Work out the finished part from the listing and answer in its coordinate system (mm). Round coordinates to 2 decimals unless told otherwise and drop trailing zeros. Loops run counter-clockwise (first coordinate to the right, second up) from the corner with the lowest first, then second, coordinate; pieces in that order, holes last. Notation, with made-up numbers: (69.25, 11.25) - (99.25, 11.25) arc R27 cw to (99.25, 27.25) - close; hole circle Ø7 at (76, 52). An arc over 180 degrees is marked (long way). Answer as CSV lines item,"result". Start each with the question number.
Q1. Section A-A on y = 7 is taken. Write down the section's boundary in (x, z), then the cut area to 3 significant figures.
Q2. This flat-tipped pin is pushed along its axis until it touches: pin 1 Ø12 at (x, y) = (17.5, 9) entering from +Z. Where does it stop, or does it pass through?
Q3. Straight lines are drawn through the part: L1, parallel to Z at x = 14, y = 11.5; L2, parallel to Z at x = 18.75, y = 9.5. For each, find the intervals that lie inside material, in ascending order. Write a range as [from, to].
```python
from build123d import *

# Parameters (mm, degrees)
SKETCH1_W           = 29
SKETCH1_H           = 125.5
BOSS_EXTRUDE1_DEPTH = 43
FILLET1_R           = 1.5


with BuildPart() as part:
    # Sketch1 → Boss-Extrude1 (new body)
    with BuildSketch(Plane(origin=(0, 0, 0), x_dir=(1, 0, 0), z_dir=(0, 1, 0))):
        with Locations((14.5, -62.75)):
            Rectangle(SKETCH1_W, SKETCH1_H)
        with BuildLine():
            Line((0, -125.5), (29, -125.5))
            ThreePointArc((29, -125.5), (14.5, -140), (0, -125.5))
        make_face()
    extrude(amount=BOSS_EXTRUDE1_DEPTH)

    # Fillet1
    fillet1_edges = [part.edges().sort_by_distance(p)[0] for p in [
        (14.5, 43, 0),
        (0, 43, 62.75),
        (14.5, 43, 140),
        (29, 43, 62.75),
        (14.5, 0, 140),
        (0, 0, 62.75),
        (14.5, 0, 0),
        (29, 0, 62.75),
        (0, 21.5, 0),
        (29, 21.5, 0),
    ]]
    fillet(fillet1_edges, radius=FILLET1_R)


solid = part.part
```
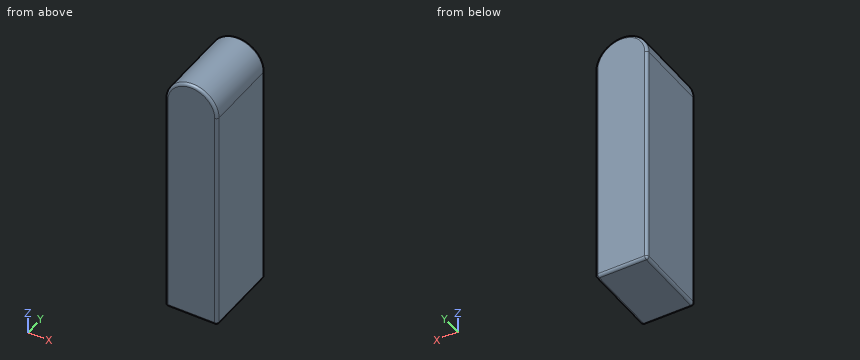
Findings:
1,outline,"(0, 1.5) arc R1.5 ccw to (1.5, 0) - (27.5, 0) arc R1.5 ccw to (29, 1.5) - (29, 125.5) arc R14.5 ccw to (0, 125.5) - close"
1,area,"3,970 mm^2"
2,pin 1,"stops at z = 140"
3,L1,"z = [0, 139.99]"
3,L2,"z = [0, 139.36]"
